from build123d import *


with BuildPart() as part:
    # Çizim1 → Döndür5 (revolve)
    with BuildSketch(Plane.XY, mode=Mode.PRIVATE) as d_nd_r5_sk:
        with BuildLine():
            Line((-62.5, 80.513349387), (-62.5, -19.486650613))
            ThreePointArc((-62.5, -19.486650613), (-57.140269015, -36.599719971), (-42.976190476, -47.598026124))
            ThreePointArc((-42.976190476, -47.598026124), (-42.267986549, -48.147941431), (-42, -49.003594899))
            Line((-42, -49.003594899), (-42, -64.486650613))
            Line((-42, -64.486650613), (-40.5, -64.486650613))
            Line((-40.5, -64.486650613), (-40.5, -58.486650613))
            Line((-40.5, -58.486650613), (-34.5, -58.486650613))
            Line((-34.5, -58.486650613), (-34.5, -54.486650613))
            Line((-34.5, -54.486650613), (-40.5, -54.486650613))
            Line((-40.5, -54.486650613), (-40.5, -47.942757163))
            ThreePointArc((-40.5, -47.942757163), (-40.782933856, -47.065973267), (-41.525, -46.519951836))
            ThreePointArc((-41.525, -46.519951836), (-55.624256745, -36.145544634), (-61, -19.486650613))
            Line((-61, -19.486650613), (-61, 80.513349387))
            Line((-61, 80.513349387), (-62.5, 80.513349387))
        make_face()
    revolve(d_nd_r5_sk.sketch.rotate(Axis((0, 0, 0), (0, 1, 0)), 270), axis=Axis((0, 0, 0), (0, 1, 0)))


solid = part.part
Geometry: final body of the model. Coordinates: model frame, mm. A direction names the side the tool comes from. Coordinates: 2 decimals unless noted, no trailing zeros. Loops run counter-clockwise (first coordinate to the right, second up) from the corner with the lowest first, then second, coordinate; pieces in that order, holes last. Notation, with made-up numbers: M -24,81.25 L 9,81.25 A28 cw 9,113.25 Z; hole C 84.25,58 d4. An arc over 180 degrees is marked long. One line per item, written item: value. Start each with the question number.
1) Cut plane D-D (y = -24). Return loops of the section in (x, z), then the cut area to 3 significant figures.
2) Cut plane C-C (y = 13). Return loops of the section in (x, z), then the cut area to 3 significant figures.
3) Cut plane B-B (z = 0). Return loops of the section in (x, y) (3 decimals), then the cut area to 3 significant figures.
4) Material intervals for L1, parallel to X at y = 29, z = 0; L2, parallel to Y at x = 32.5, z = 18; L3, parallel to Z at x = 27.5, y = -39, sorted ascending. Write a range as from..to.
5) Reachability of faces 1 (the cylindrical face through (-34.15, -51.17, -21.77)), 2 (the cylindrical face through (-34.15, -61.44, -21.77)), 3 (the flat face through (60, 80.513, 14)) from +Z, -Z, +X, -X, +Y, -Y: full face, straight path, thin tool, end or side. Return the list, or none.
6) Pin query (flat end, axial travel): P1, Ø10, axis at x = -23.5, z = 33.5, coming from the +Y side; P2, Ø3, axis at x = -21, y = 53.5, coming from the +Z side; P3, Ø4, axis at x = 3, y = -39.5, coming from the -Z side. Return the tip coordinate at first contact, or that it passes through.
7) Draft query along X for faces 4 (the cylindrical face through (-12.62, -56.85, -40.06)), 5 (the cylindrical face through (59.55, 31.21, 13.22)), 6 (the flat face through (-18, -58.487, -30)), 7 (the flat face through (-22, -64.487, 34.4)). Return one class per face: released by +X, released by -X, zero draft, split by the parting line, or undercut.
8) Cut plane A-A (x = 0). Return loops of the section in (y, z) (3 decimals), then the cut area to 3 significant figures.
Evaluation:
1. outline: C 0,0 d124.32; hole C 0,0 d121.28
1. area: 586 mm^2
2. outline: C 0,0 d125; hole C 0,0 d122
2. area: 582 mm^2
3. outline: M -62.5,-19.487 A30 ccw -42.976,-47.598 A1.5 cw -42,-49.004 L -42,-64.487 L -40.5,-64.487 L -40.5,-58.487 L -34.5,-58.487 L -34.5,-54.487 L -40.5,-54.487 L -40.5,-47.943 A1.5 ccw -41.525,-46.52 A28.5 cw -61,-19.487 L -61,80.513 L -62.5,80.513 Z; M 34.5,-58.487 L 40.5,-58.487 L 40.5,-64.487 L 42,-64.487 L 42,-49.004 A1.5 cw 42.976,-47.598 A30 ccw 62.5,-19.487 L 62.5,80.513 L 61,80.513 L 61,-19.487 A28.5 cw 41.525,-46.52 A1.5 ccw 40.5,-47.943 L 40.5,-54.487 L 34.5,-54.487 Z
3. area: 510 mm^2
4. L1: -62.5..-61, 61..62.5
4. L2: -58.49..-54.49
4. L3: -47.96..-45.63, 45.63..47.96
5. face 1: +Y
5. face 2: -Y
5. face 3: +Z, -Z, +X, -X, +Y
6. P1: y = -44.63
6. P2: z = 59.38
6. P3: z = -56.41
7. face 4: split by the parting line
7. face 5: undercut
7. face 6: undercut
7. face 7: zero draft
8. outline: M -64.487,-42 L -49.004,-42 A1.5 cw -47.598,-42.976 A30 ccw -19.487,-62.5 L 80.513,-62.5 L 80.513,-61 L -19.487,-61 A28.5 cw -46.52,-41.525 A1.5 ccw -47.943,-40.5 L -54.487,-40.5 L -54.487,-34.5 L -58.487,-34.5 L -58.487,-40.5 L -64.487,-40.5 Z; M -64.487,40.5 L -58.487,40.5 L -58.487,34.5 L -54.487,34.5 L -54.487,40.5 L -47.943,40.5 A1.5 ccw -46.52,41.525 A28.5 cw -19.487,61 L 80.513,61 L 80.513,62.5 L -19.487,62.5 A30 ccw -47.598,42.976 A1.5 cw -49.004,42 L -64.487,42 Z
8. area: 510 mm^2
